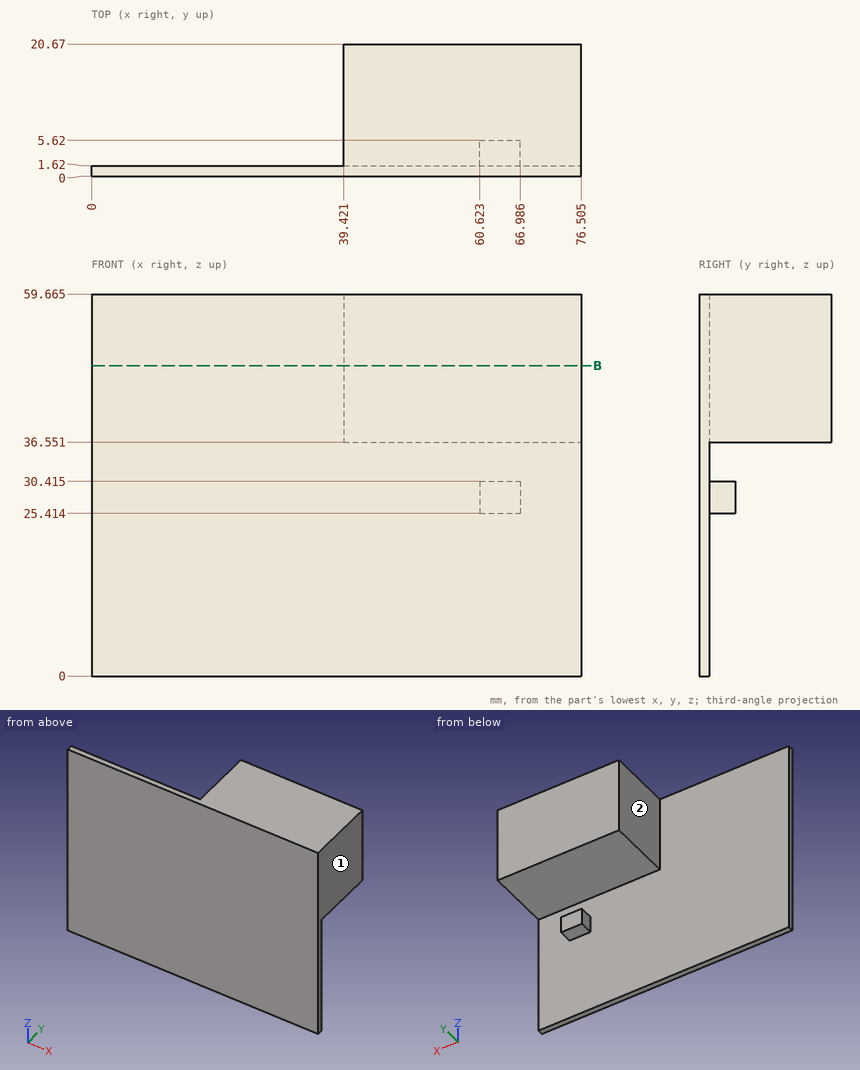
The drawing under review shows one solid part. Ordinate dimensions are in mm from its lowest x, y, z. A direction names the side the tool comes from. Coordinates: 2 decimals unless noted, no trailing zeros. Order: outer loops, then holes, each group sorted by start corner. A loop starts at its lowest first (then second) coordinate and runs counter-clockwise, first axis right, second up. Notation, with made-up numbers: (-35.5, 56.5) - (-30.5, 56.5) arc R13 ccw to (-30.5, 63.5) - close; hole circle Ø6 at (84, 46.25). An arc over 180 degrees is marked (long way). Put each result on its own line as item: value.
1) Insertion check: P1, Ø4, axis at x = 64, z = 27.5, coming from the +Y side; P2, Ø4, axis at x = 10, y = 3, coming from the -Z side; P3, Ø3, axis at y = 4, z = 27, coming from the +X side; P4, Ø4, axis at x = 47.5, z = 17, coming from the +Y side. Each pin has a flat end and moves straight along its axis. Give the tip position at first contact, or say it passes through.
Response values:
P1: stops at y = 5.62
P2: stops at z = 0
P3: stops at x = 66.99
P4: stops at y = 1.62
2) Take a section at B-B, the plane z = 48.5. Give the boundary of the cut face in (x, y) (1 decimal).
Response values:
outline: (0, 0) - (76.5, 0) - (76.5, 20.7) - (39.4, 20.7) - (39.4, 1.6) - (0, 1.6) - close
3) Tool access review of the marked faces 1 and 2: name each direction out of +Z, -Z, +X, -X, +Y, -Y from which nothing blocks a thin tool from reaching the whole face with its end or side.
Response values:
face 1: +Z, -Z, +X, +Y, -Y
face 2: +Z, -Z, -X, +Y
4) Wall thickness on L1, parallel to Y at x = 60.5, z = 23; L2, parallel to X at y = 10.5, z = 43.5 (1 decimal); L3, parallel to Y at x = 66.5, z = 29.5: over which ranges is each line inside the solid? List them lowest first. Write a range as from..to.
Response values:
L1: y = 0..1.62
L2: x = 39.4..76.5
L3: y = 0..5.62
